Design review of the part built by this model. Coordinates are the model's own, in mm. A direction names the side the tool comes from. Coordinates: 2 decimals unless noted, no trailing zeros. Loops run counter-clockwise (first coordinate to the right, second up) from the corner with the lowest first, then second, coordinate; pieces in that order, holes last. Notation, with made-up numbers: M 50.25,-5 L 70.25,-5 A18 ccw 70.25,8 Z; hole C 2.25,-5.5 d4. An arc over 180 degrees is marked long. One line per item, written item: value.
```python
from build123d import *

# Parameters (mm, degrees)
SKETCH6_W           = 15
SKETCH6_H           = 6
SKETCH8_W           = 10
SKETCH8_H           = 12
BOSS_EXTRUDE2_DEPTH = 9
SKETCH9_W           = 1
SKETCH9_H           = 12
CUT_EXTRUDE2_DEPTH  = 15
SKETCH10_R          = 1.95
BOSS_EXTRUDE3_DEPTH = 0.9
SKETCH11_R          = 1.5
BOSS_EXTRUDE4_DEPTH = 8.67
SKETCH12_W          = 2.491987158
SKETCH12_H          = 0.5
CUT_EXTRUDE3_DEPTH  = 8.67
SKETCH13_R          = 2.5
SKETCH13_W          = 1.5
SKETCH13_H          = 0.3
BOSS_EXTRUDE5_DEPTH = 2


with BuildPart() as part:
    # Sketch6 → Revolve-Thin2 (revolve)
    with BuildSketch(Plane(origin=(0, 0, 0), x_dir=(1, 0, 0), z_dir=(0, 1, 0)), mode=Mode.PRIVATE) as revolve_thin2_sk:
        with Locations((7.5, 3)):
            Rectangle(SKETCH6_W, SKETCH6_H)
    revolve(revolve_thin2_sk.sketch.rotate(Axis((0, 0, 0), (1, 0, 0)), 180), axis=Axis((0, 0, 0), (1, 0, 0)))

    # Sketch8 → Boss-Extrude2 (add)
    with BuildSketch(Plane.ZY):
        Rectangle(SKETCH8_W, SKETCH8_H)
    extrude(amount=BOSS_EXTRUDE2_DEPTH)

    # Sketch9 → Cut-Extrude2 (cut)
    with BuildSketch(Plane.ZY):
        with Locations((5.5, 0)):
            Rectangle(SKETCH9_W, SKETCH9_H)
        with Locations((-5.5, 0)):
            Rectangle(SKETCH9_W, SKETCH9_H)
    extrude(amount=-CUT_EXTRUDE2_DEPTH, mode=Mode.SUBTRACT)

    # Sketch10 → Boss-Extrude3 (add)
    with BuildSketch(Plane.ZY.offset(9)):
        with Locations(Location((0, 0, 0), (0, 0, 180))):
            Circle(SKETCH10_R)
    extrude(amount=BOSS_EXTRUDE3_DEPTH)

    # Sketch11 → Boss-Extrude4 (add)
    with BuildSketch(Plane.ZY.offset(9.9)):
        Circle(SKETCH11_R)
    extrude(amount=BOSS_EXTRUDE4_DEPTH)

    # Sketch12 → Cut-Extrude3 (cut)
    with BuildSketch(Plane.ZY.offset(18.57)):
        with Locations((0, 1.25)):
            Rectangle(SKETCH12_W, SKETCH12_H)
    extrude(amount=-CUT_EXTRUDE3_DEPTH, mode=Mode.SUBTRACT)

    # Sketch13 → Boss-Extrude5 (add)
    with BuildSketch(Plane(origin=(15, 0, 0), x_dir=(0, 0, -1), z_dir=(1, 0, 0))):
        with Locations(Location((0, 0, 0), (0, 0, 180))):
            Circle(SKETCH13_R)
        with Locations((0, 3.5)):
            Rectangle(SKETCH13_W, SKETCH13_H)
        with Locations((0, -3.5)):
            Rectangle(SKETCH13_W, SKETCH13_H)
    extrude(amount=BOSS_EXTRUDE5_DEPTH)


solid = part.part
```
(1) To check wall thickness, follow line 1 along X through (y, z) = (-4.5, 1); line 2 along X through (y, z) = (0.5, 1.5); line 3 along Y through (x, z) = (1.5, -2.5). State the ranges of each line that lie inside material, in increasing order. Write a range as [from, to].
Reply:
line 1: x = [-9, 15]
line 2: x = [-9.9, 17]
line 3: y = [-5.45, 5.45]
(2) We need section D-D on y = 0. State the section outline as (x, z) points, then the cut area to 3 significant figures.
Reply:
outline: M -18.57,-1.5 L -9.9,-1.5 L -9.9,-1.95 L -9,-1.95 L -9,-5 L 15,-5 L 15,-2.5 L 17,-2.5 L 17,2.5 L 15,2.5 L 15,5 L -9,5 L -9,1.95 L -9.9,1.95 L -9.9,1.5 L -18.57,1.5 Z
area: 280 mm2
(3) Tool access review of faces 1 (the cylindrical face through (16, -0.1, -2.5)), 2 (the flat face through (0, 5, -4)), 3 (the flat face through (16, 3.65, 0)), 4 (the flat face through (16, 3.35, 0)), 5 (the flat face through (-9.9, 1.3, 0)): name each direction out of +Z, -Z, +X, -X, +Y, -Y from which nothing blocks a thin tool from reaching the whole face with its end or side.
Reply:
face 1: +X
face 2: -Z, +X, +Y
face 3: +Z, -Z, +X, +Y
face 4: +Z, -Z, +X
face 5: -X
(4) We need section C-C on x = 2.5. State the section outline as (y, z) points, then the cut area to 3 significant figures.
Reply:
outline: M -3.32,-5 L 3.32,-5 A6 ccw 3.32,5 L -3.32,5 A6 ccw Z
area: 104 mm2
(5) We need section A-A on y = 5. State the section outline as (x, z) points.
Reply:
outline: M -9,-5 L 0,-5 L 0,-3.32 L 15,-3.32 L 15,3.32 L 0,3.32 L 0,5 L -9,5 Z
(6) We need section B-B on z = 3.5. State the section outline as (x, y) points, then the cut area to 3 significant figures.
Reply:
outline: M -9,-6 L 0,-6 L 0,-4.87 L 15,-4.87 L 15,4.87 L 0,4.87 L 0,6 L -9,6 Z
area: 254 mm2
(7) Insertion check: pin 1 (1.3 mm diameter, centred on y = -5.5, z = 3, fed in from +X); pin 2 (1.5 mm diameter, centred on y = -4.5, z = 1, fed in from -X); pin 3 (1.5 mm diameter, centred on y = 2.5, z = -0.5, fed in from -X). Each pin has a flat end and moves straight along its axis. Give the tip position at first contact, or say it passes through.
Reply:
pin 1: stops at x = 15
pin 2: stops at x = -9
pin 3: stops at x = -9.9
